The model under review builds one solid part; all positions refer to its coordinate system, in mm. Face numbers are marked on the shaded views. A direction names the side the tool comes from. Coordinates: 2 decimals unless noted, no trailing zeros. Order: outer loops, then holes, each group sorted by start corner. A loop starts at its lowest first (then second) coordinate and runs counter-clockwise, first axis right, second up.
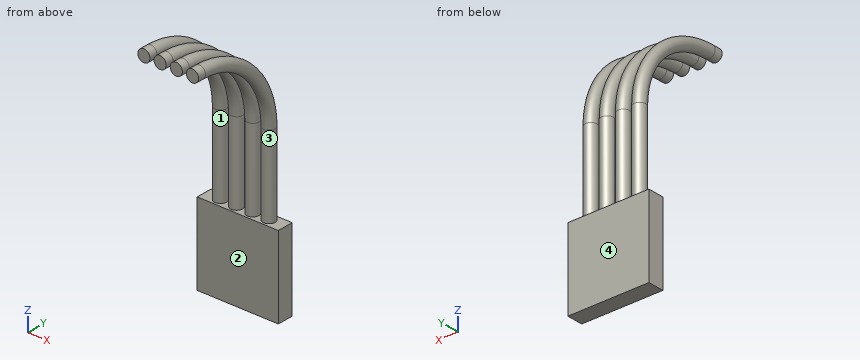
from build123d import *

# Parameters (mm, degrees)
SKIZZE1_W                       = 10
SKIZZE1_H                       = 2
AUFSATZ_LINEAR_AUSTRAGEN1_DEPTH = 10
SKIZZE2_R                       = 0.75
AUFSATZ_LINEAR_AUSTRAGEN2_DEPTH = 10
SKIZZE4_R                       = 0.75
LINEARES_MUSTER1_COUNT          = 4
LINEARES_MUSTER1_PITCH          = 2


with BuildPart() as part:
    # Skizze1 → Aufsatz-Linear austragen1 (new body)
    with BuildSketch(Plane.XY):
        Rectangle(SKIZZE1_W, SKIZZE1_H)
    extrude(amount=AUFSATZ_LINEAR_AUSTRAGEN1_DEPTH)

    # Skizze2 → Aufsatz-Linear austragen2 (add)
    with BuildSketch(Plane.XY.offset(10)):
        with Locations(Location((-1, 0, 0), (0, 0, 180))):
            Circle(SKIZZE2_R)
        with Locations(Location((-3, 0, 0), (0, 0, 180))):
            Circle(SKIZZE2_R)
        with Locations(Location((1, 0, 0), (0, 0, 180))):
            Circle(SKIZZE2_R)
        with Locations(Location((3, 0, 0), (0, 0, 180))):
            Circle(SKIZZE2_R)
    extrude(amount=AUFSATZ_LINEAR_AUSTRAGEN2_DEPTH)

    # Austragung1: sweep along a path in Skizze3
    with BuildLine(Plane(origin=(-3, 0, 0), x_dir=(0, 0, -1), z_dir=(1, 0, 0))) as austragung1_path:
        Line((-30, -11), (-30, -10))
        ThreePointArc((-30, -10), (-27.071067812, -2.928932188), (-20, 0))
    # Skizze4 → Austragung1 (sweep)
    with BuildSketch(Plane.XY.offset(20)):
        with Locations((-3, 0)):
            Circle(SKIZZE4_R)
    austragung1 = sweep(path=austragung1_path.line)

    # Lineares Muster1: Austragung1 ×4
    with Locations(*[(i * LINEARES_MUSTER1_PITCH, 0, 0) for i in range(1, LINEARES_MUSTER1_COUNT)]):
        add(austragung1)


solid = part.part
(1) Consider section A-A (z = 12). Give the boundary of the cut face in (x, y).
(2) Tool access review of the marked faces 3 and 4: name each direction out of +Z, -Z, +X, -X, +Y, -Y from which nothing blocks a thin tool from reaching the whole face with its end or side.
(3) Insertion check: pin 1 Ø2 at (x, y) = (2.5, -2.5) entering from -Z; pin 2 Ø1 at (x, z) = (3, 17) entering from -Y; pin 3 Ø2 at (x, y) = (0, -5.5) entering from -Z. Each pin has a flat end and moves straight along its axis. Give the tip position at first contact, or say it passes through.
(4) Wall thickness on line 1 (X direction, y = -3.5, z = 27); line 2 (X direction, y = 0, z = 21.5); line 3 (Y direction, x = 0.5, z = 6): over which ranges is each line inside the solid? List them lowest first.
(5) Consider section B-B (x = -1). Give the boundary of the cut face in (y, z), then the cut area to 3 significant figures.
(6) Consider section C-C (z = 2). Give the boundary of the cut face in (x, y).
(7) The part is to be moulded in two halves that separate along X. For the marked faces 1 and 2, say which applies: +X half, -X half, draft (parallel to the pull), parting line (faces both ways), or undercut.
(8) Consider section D-D (y = -4). Give the number of separate pieces and of enclosed holes in the cut face, then the cut area to 3 significant figures.
Findings:
1. outline: circle Ø1.5 at (-3, 0); circle Ø1.5 at (-1, 0); circle Ø1.5 at (1, 0); circle Ø1.5 at (3, 0)
2. face 3: none
2. face 4: +Z, -Z, +X, -X, +Y
3. pin 1: stops at z = 23.82
3. pin 2: stops at y = -0.75
3. pin 3: stops at z = 27.71
4. line 1: x = -3.6 to -2.4, -1.6 to -0.4, 0.4 to 1.6, 2.4 to 3.6
4. line 2: x = -3.74 to -2.26, -1.74 to -0.26, 0.26 to 1.74, 2.26 to 3.74
4. line 3: y = -1 to 1
5. outline: (-11, 29.25) - (-10, 29.25) arc R9.25 cw to (-0.75, 20) - (-0.75, 10) - (-1, 10) - (-1, 0) - (1, 0) - (1, 10) - (0.75, 10) - (0.75, 20) arc R10.75 ccw to (-10, 30.75) - (-11, 30.75) - close
5. area: 60.1 mm2
6. outline: (-5, -1) - (5, -1) - (5, 1) - (-5, 1) - close
7. face 1: undercut
7. face 2: draft
8. separate pieces: 4
8. enclosed holes: 0
8. area: 8.85 mm2
